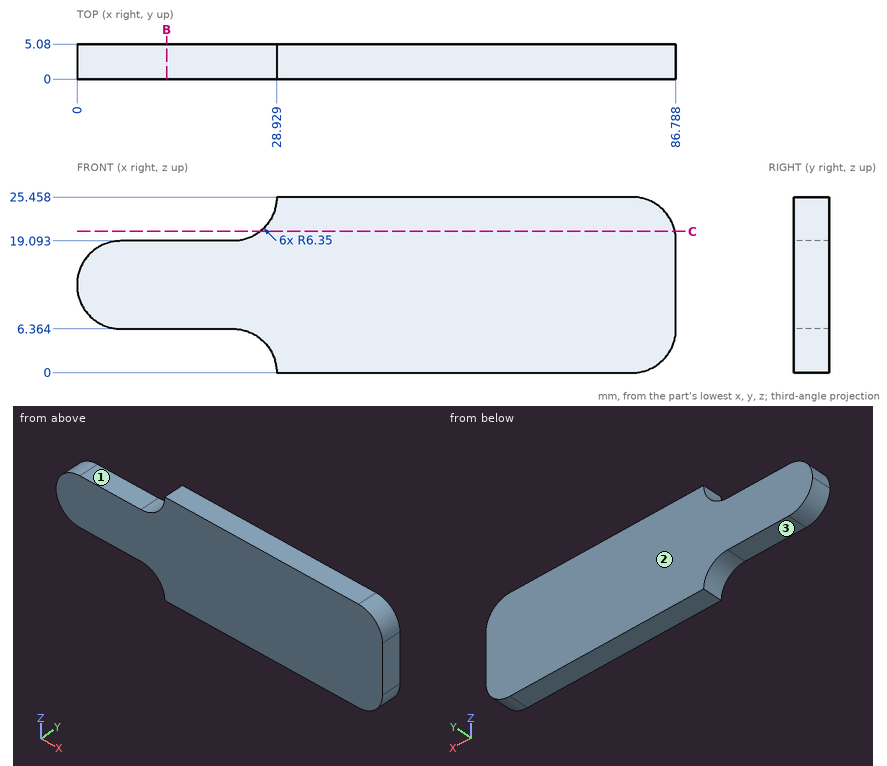
For this review, use the dimensioned drawing (mm, ordinates from the lowest corner) and the shaded views. A direction names the side the tool comes from. Round coordinates to 2 decimals unless told otherwise and drop trailing zeros. Order: outer loops, then holes, each group sorted by start corner. A loop starts at its lowest first (then second) coordinate and runs counter-clockwise, first axis right, second up. Notation, with made-up numbers: M -12.5,19.5 L 13.5,19.5 A23 ccw 13.5,49.5 Z; hole C -30,-29.5 d7. An arc over 180 degrees is marked long. Write each question's results on one line, items separated by ' | '. Start each with the question number.
1. To check wall thickness, follow L1, parallel to Z at x = 14.5, y = 4 (1 decimal); L2, parallel to Z at x = 25.5, y = 3.9 (1 decimal); L3, parallel to X at y = 3.05, z = 11.5. State the ranges of each line that lie inside material, in increasing order. Write a range as [from, to].
2. Add section B-B (x = 13). State the section outline as (y, z) points (1 decimal).
3. Clearance check with flat-ended pins moving along their axes: pin 1 Ø1.5 at (x, y) = (15.5, 3.5) entering from +Z; pin 2 Ø1.5 at (x, y) = (16.5, 2) entering from -Z. State where each tip first meets the part, or that it passes through.
4. Add section C-C (z = 20.5). State the section outline as (x, y) points (1 decimal).
5. Tool access review of the marked faces 1, 2 and 3: name each direction out of +Z, -Z, +X, -X, +Y, -Y from which nothing blocks a thin tool from reaching the whole face with its end or side.
Output values:
1) L1: [6.4, 19.1] | L2: [5.7, 19.8] | L3: [0.12, 86.79]
2) outline: M 0,6.4 L 5.1,6.4 L 5.1,19.1 L 0,19.1 Z
3) pin 1: z = 19.09 | pin 2: z = 6.36
4) outline: M 26.6,0 L 86.6,0 L 86.6,5.1 L 26.6,5.1 Z
5) face 1: +Z, -X, +Y, -Y | face 2: +Z, -Z, +X, -X, +Y | face 3: -Z, -X, +Y, -Y
